Geometry check sheet. Reference: drawing and pictorial views, mm from the part's lowest x, y, z. Give positions to 0.01 mm unless a question says otherwise; leave off trailing zeros. Order: outer loops, then holes, each group sorted by start corner. A loop starts at its lowest first (then second) coordinate and runs counter-clockwise, first axis right, second up. Notation, with made-up numbers: (36.5, 89) - (71.5, 89) arc R27 ccw to (71.5, 113) - close; hole circle Ø1 at (21, 10). An arc over 180 degrees is marked (long way). Answer as a JSON object with one key per item and string values.
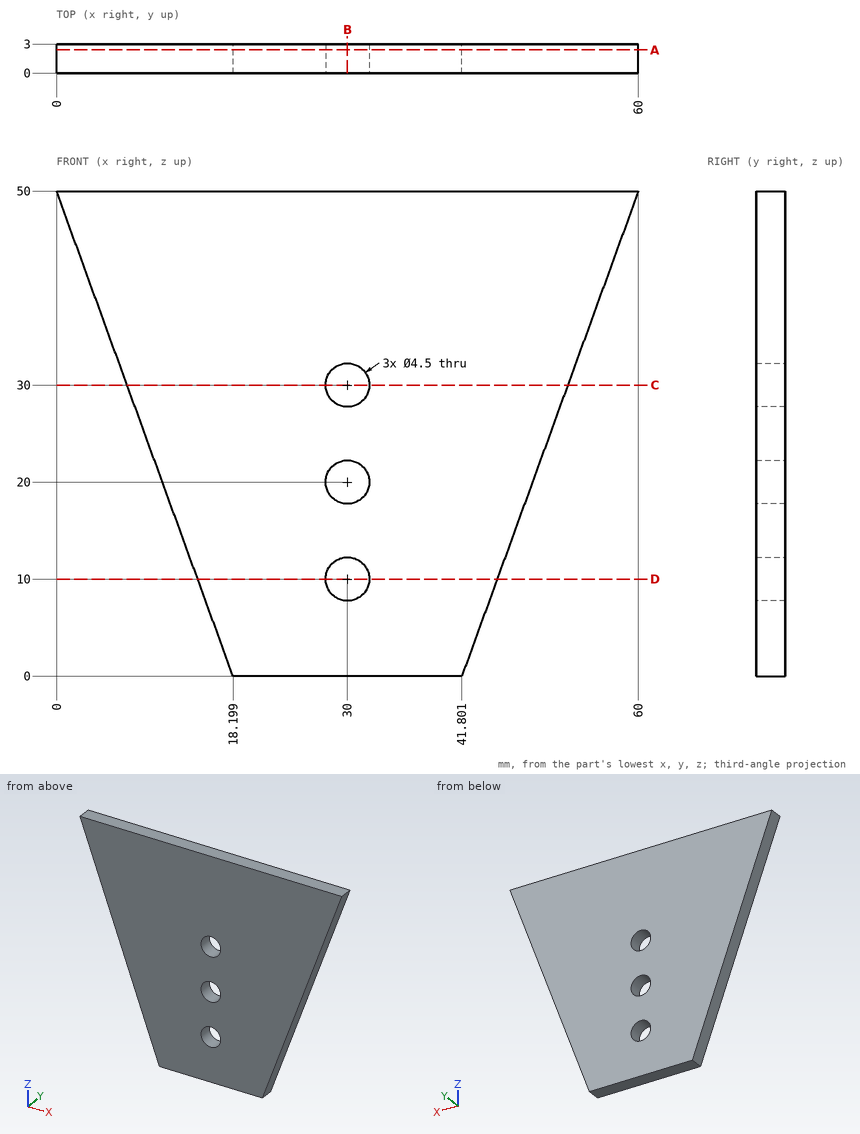
(1) Gauge pin test, flat end, axial feed: pin 1 Ø2 at (x, z) = (11, 13) entering from +Y. Record the tip position at first contact, or that the pin passes through.
Computed values:
{"pin 1": "passes through"}
(2) Section check C-C (z = 30). Record the cut outline in (x, y).
Computed values:
{"outline": "(7.28, 0) - (27.75, 0) - (27.75, 3) - (7.28, 3) - close; (32.25, 0) - (52.72, 0) - (52.72, 3) - (32.25, 3) - close"}
(3) Section check B-B (x = 30). Record the cut outline in (y, z).
Computed values:
{"outline": "(0, 0) - (3, 0) - (3, 7.75) - (0, 7.75) - close; (0, 12.25) - (3, 12.25) - (3, 17.75) - (0, 17.75) - close; (0, 22.25) - (3, 22.25) - (3, 27.75) - (0, 27.75) - close; (0, 32.25) - (3, 32.25) - (3, 50) - (0, 50) - close"}
(4) Section check A-A (y = 2.4). Record the cut outline in (x, z).
Computed values:
{"outline": "(0, 50) - (18.2, 0) - (41.8, 0) - (60, 50) - close; hole circle Ø4.5 at (30, 10); hole circle Ø4.5 at (30, 20); hole circle Ø4.5 at (30, 30)"}
(5) Material ranges on line 1 along X through (y, z) = (1.4, 20); line 2 along X through (y, z) = (0.7, 30); line 3 along X through (y, z) = (2.8, 40.5), recorded low to high. Write a range as [from, to].
Computed values:
{"line 1": "x = [10.92, 27.75], [32.25, 49.08]", "line 2": "x = [7.28, 27.75], [32.25, 52.72]", "line 3": "x = [3.46, 56.54]"}
(6) Section check D-D (z = 10). Record the cut outline in (x, y).
Computed values:
{"outline": "(14.56, 0) - (27.75, 0) - (27.75, 3) - (14.56, 3) - close; (32.25, 0) - (45.44, 0) - (45.44, 3) - (32.25, 3) - close"}
